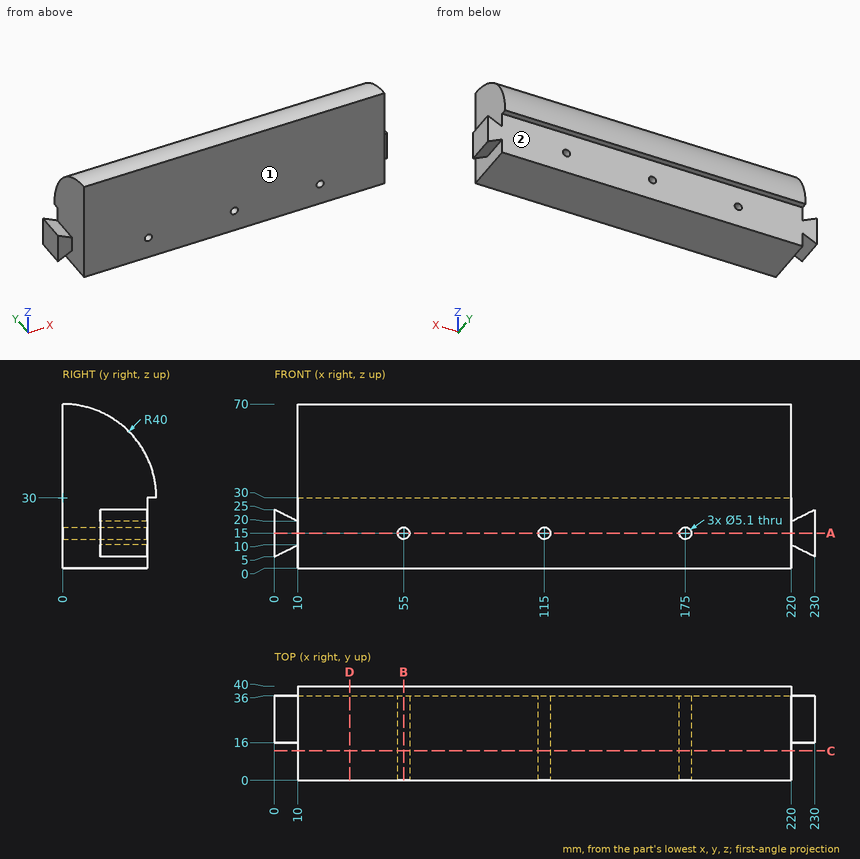
For this review, use the dimensioned drawing (mm, ordinates from the lowest corner) and the shaded views. A direction names the side the tool comes from. Coordinates: 2 decimals unless noted, no trailing zeros. Order: outer loops, then holes, each group sorted by start corner. A loop starts at its lowest first (then second) coordinate and runs counter-clockwise, first axis right, second up. Notation, with made-up numbers: (51, -36.75) - (108, -36.75) arc R18 ccw to (108, -27.75) - close; hole circle Ø9 at (-36, 87.5). An arc over 180 degrees is marked (long way). Use one line per item in the form item = value.
Q1. Consider section A-A (z = 15). Give the boundary of the cut face in (x, y).
Checked values:
outline = (0, 16) - (10, 16) - (10, 0) - (52.45, 0) - (52.45, 36) - (0, 36) - close; (57.55, 0) - (112.45, 0) - (112.45, 36) - (57.55, 36) - close; (117.55, 0) - (172.45, 0) - (172.45, 36) - (117.55, 36) - close; (177.55, 0) - (220, 0) - (220, 16) - (230, 16) - (230, 36) - (177.55, 36) - close
Q2. Consider section D-D (x = 32). Give the boundary of the cut face in (y, z).
Checked values:
outline = (0, 0) - (36, 0) - (36, 30) - (40, 30) arc R40 ccw to (0, 70) - close
Q3. Consider section B-B (x = 55). Give the boundary of the cut face in (y, z), then the cut area to 3 significant figures.
Checked values:
outline = (0, 0) - (36, 0) - (36, 12.45) - (0, 12.45) - close; (0, 17.55) - (36, 17.55) - (36, 30) - (40, 30) arc R40 ccw to (0, 70) - close
area = 2,150 mm2
Q4. For probe 1 along X at (y, z) = (13, 15); probe 2 along X at (y, z) = (24, 15); probe 3 along X at (y, z) = (29, 29), list the stretches that pass through material, from the lowest coordinate up. Write a range as from..to.
Checked values:
probe_1 = 10..52.45, 57.55..112.45, 117.55..172.45, 177.55..220
probe_2 = 0..52.45, 57.55..112.45, 117.55..172.45, 177.55..230
probe_3 = 10..220
Q5. For P1, Ø2, axis at x = 181, y = 27.5, coming from the +Z side; P2, Ø8, axis at x = 115, z = 15, coming from the +Y side; P3, Ø12, axis at y = 26.5, z = 42.5, coming from the +X side, all flat-tipped, find the tip position at first contact; note any pin that passes through.
Checked values:
P1 = 59.96
P2 = 36
P3 = 220
Q6. For the marked faces 1 and 2, list the 3-axis set-ups (+Z, -Z, +X, -X, +Y, -Y) from which the entire face can be reached by the end or side of a thin tool; tool diameter is ignored.
Checked values:
face_1 = +Z, -Z, +X, -X, -Y
face_2 = -Z, +X, -X, +Y
Q7. Consider section C-C (y = 12.5). Give the boundary of the cut face in (x, z), then the cut area to 3 significant figures.
Checked values:
outline = (10, 0) - (220, 0) - (220, 68) - (10, 68) - close; hole circle Ø5.1 at (55, 15); hole circle Ø5.1 at (115, 15); hole circle Ø5.1 at (175, 15)
area = 14,200 mm2
